Autodesk Inventor part; units mm, degrees
ref_plane "YZ Plane" through (0, 0, 0) normal (1, 0, 0) x (0, 1, 0)
ref_plane "XZ Plane" through (0, 0, 0) normal (0, 1, 0) x (-1, 0, 0)
ref_plane "XY Plane" through (0, 0, 0) normal (0, 0, 1) x (1, 0, 0)
sketch "Sketch1" plane through (0, 0, 0) normal (0, 0, 1) x (1, 0, 0)
  line L0 (84.9408, 79.3264) -> (123.4503, 45.7166)
  line L1 (168.5483, 110.2412) -> (161.1682, 59.6633)
  line L2 (90.9184, 92.6811) -> (125.2091, 88.4019)
  line L3 (132.0626, 90.936) -> (155.3205, 116.4945)
  arc A0 (90.9184, 92.6811) -> (84.9408, 79.3264) centre (89.9711, 85.09) ccw
  arc A1 (128.9448, 88.8334) -> (132.0626, 90.936) centre (126.192, 96.2783) ccw
  arc A2 (125.2091, 88.4019) -> (128.9448, 88.8334) centre (126.192, 96.2783) ccw
  arc A3 (123.4503, 45.7166) -> (161.1682, 59.6633) centre (138.5082, 62.9697) ccw
  arc A4 (168.5483, 110.2412) -> (155.3205, 116.4945) centre (160.9785, 111.3458) ccw
  line L4 (84.1057, 78.3696) -> (122.6152, 44.7598)
  arc A5 (122.6152, 44.7598) -> (162.4249, 59.4799) centre (138.5082, 62.9697) ccw
  line L5 (162.4249, 59.4799) -> (169.805, 110.0578)
  arc A6 (169.805, 110.0578) -> (154.3812, 117.3492) centre (160.9785, 111.3458) ccw
  line L6 (154.3812, 117.3492) -> (131.1233, 91.7908)
  arc A7 (128.5043, 90.0246) -> (131.1233, 91.7908) centre (126.192, 96.2783) ccw
  arc A8 (125.3663, 89.6621) -> (128.5043, 90.0246) centre (126.192, 96.2783) ccw
  line L7 (125.3663, 89.6621) -> (91.0757, 93.9413)
  arc A9 (91.0757, 93.9413) -> (84.1057, 78.3696) centre (89.9711, 85.09) ccw
  point P0 (0, 0)
  dimension "d1" = 1.27
extrude "Extrusion1" add sketch "Sketch1" along normal blind 9
ref_plane "Work Plane1" through (0, 0, 4.5) normal (0, 0, 1) x (1, 0, 0)
properties part number "290 mm Belt"
The model under review builds one solid part; all positions refer to its coordinate system, in mm. A direction names the side the tool comes from. Give positions to 0.01 mm unless a question says otherwise; leave off trailing zeros. Order: outer loops, then holes, each group sorted by start corner. A loop starts at its lowest first (then second) coordinate and runs counter-clockwise, first axis right, second up. Notation, with made-up numbers: (-16, 6) - (-5, 6) arc R20 cw to (-5, 19) - close; hole circle Ø4 at (27, -7). An arc over 180 degrees is marked (long way). Use CSV: the item, a comma, the result in double quotes. Start each with the question number.
Q1. Clearance check with flat-ended pins moving along their axes: pin 1 Ø2 at (x, z) = (132.5, 6) entering from +Y; pin 2 Ø1.5 at (x, z) = (135, 7) entering from -Y. State where each tip first meets the part, or that it passes through.
Q2. To check wall thickness, follow line 1 along Y through (x, z) = (130.5, 2); line 2 along X through (y, z) = (61.5, 0.5); line 3 along X through (y, z) = (55, 2.5). State the ranges of each line that lie inside material, in increasing order. Write a range as [from, to].
Q3. We need section A-A, the plane z = 7. Write out the cut boundary in (x, y) (1 decimal).
Q4. Tool access review of faces 5 (the cylindrical face through (127.129, 88.396, 4.437)), 6 (the cylindrical face through (129.938, 90.763, 4.437)), 7 (the flat face through (103.09, 61.8, 4.44)): name each direction out of +Z, -Z, +X, -X, +Y, -Y from which nothing blocks a thin tool from reaching the whole face with its end or side.
Q5. We need section B-B, the plane x = 153. Write out the cut boundary in (y, z), and give its area (3 significant figures).
Q6. We need section C-C, the plane y = 99. Write out the cut boundary in (x, z).
Q7. The part is to be moulded in two halves that separate along Y. For faces 1 (the flat face through (107.82, 90.57, 4.44)), 2 (the cylindrical face through (164.12, 118.32, 4.44)), 3 (the flat face through (132, 92, 9)), 4 (the flat face through (142.915, 104.749, 4.437)), say which applies: +Y half, -Y half, draft (parallel to the pull), parting line (faces both ways), or undercut.
Outcome:
1,pin 1,"stops at y = 94.4"
1,pin 2,"stops at y = 38.96"
2,line 1,"y = [40.16, 41.52], [89.61, 91.19]"
2,line 2,"x = [103.43, 105.37], [161.44, 162.72]"
2,line 3,"x = [110.88, 112.81], [159.98, 161.33]"
3,outline,"(84.1, 78.4) - (122.6, 44.8) arc R24.2 ccw to (162.4, 59.5) - (169.8, 110.1) arc R8.9 ccw to (154.4, 117.3) - (131.1, 91.8) arc R6.7 cw to (128.5, 90) arc R6.7 cw to (125.4, 89.7) - (91.1, 93.9) arc R8.9 ccw to start; hole (84.9, 79.3) - (123.5, 45.7) arc R22.9 ccw to (161.2, 59.7) - (168.5, 110.2) arc R7.6 ccw to (155.3, 116.5) - (132.1, 90.9) arc R7.9 cw to (128.9, 88.8) arc R7.9 cw to (125.2, 88.4) - (90.9, 92.7) arc R7.7 ccw to start"
4,face 5,"+Z, -Z"
4,face 6,"+Z, -Z, +Y"
4,face 7,"+Z, -Z, -X, -Y"
5,outline,"(43.63, 0) - (45.24, 0) - (45.24, 9) - (43.63, 9) - close; (113.94, 0) - (115.83, 0) - (115.83, 9) - (113.94, 9) - close"
5,area,"31.5 mm^2"
6,outline,"(137.68, 0) - (139.4, 0) - (139.4, 9) - (137.68, 9) - close; (166.91, 0) - (168.19, 0) - (168.19, 9) - (166.91, 9) - close"
7,face 1,"undercut"
7,face 2,"undercut"
7,face 3,"draft"
7,face 4,"+Y half"
